```python
from build123d import *

# Parameters (mm, degrees)
SKETCH1_W           = 145
SKETCH1_H           = 43
BOSS_EXTRUDE1_DEPTH = 30
SKETCH2_R           = 3
BOSS_EXTRUDE2_DEPTH = 30


with BuildPart() as part:
    # Sketch1 → Boss-Extrude1 (new body)
    with BuildSketch(Plane(origin=(0, 0, 0), x_dir=(1, 0, 0), z_dir=(0, 1, 0))):
        Rectangle(SKETCH1_W, SKETCH1_H)
    extrude(amount=BOSS_EXTRUDE1_DEPTH)

    # Sketch2 → Boss-Extrude2 (add)
    with BuildSketch(Plane(origin=(72.5, 0, 0), x_dir=(0, 0, -1), z_dir=(1, 0, 0))):
        with Locations((18.5, 25)):
            Circle(SKETCH2_R)
        with Locations((18.5, 5)):
            Circle(SKETCH2_R)
    extrude(amount=BOSS_EXTRUDE2_DEPTH)


solid = part.part
```
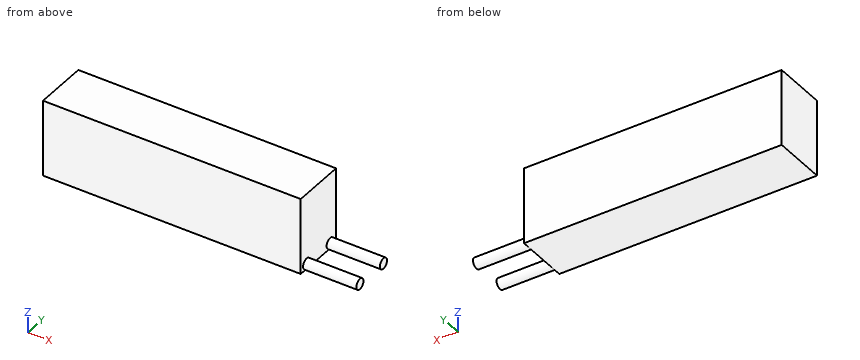
Input: part model. Units: mm. Frame: model coordinates. Give positions to 0.01 mm unless a question says otherwise; leave off trailing zeros. Order: outer loops, then holes, each group sorted by start corner. A loop starts at its lowest first (then second) coordinate and runs counter-clockwise, first axis right, second up. Notation, with made-up numbers: M 7.25,79 L 35.25,79 A21 cw 35.25,85 Z; hole C 11,70 d2. An arc over 180 degrees is marked long. Return JSON: item names as keys, results as strings.
Item 1: First-contact query: P1, Ø12, axis at x = 81, z = -13.5, coming from the -Y side. Flat tip, straight axial feed; report the tip coordinate or a pass-through.
Solutions:
{"P1": "y = 2"}
Item 2: Ray query, probe 1 along X at (y, z) = (15.25, 0); probe 2 along Z at (x, y) = (75, 27). Return the intervals inside material, ascending.
Solutions:
{"probe 1": "-72.5 to 72.5", "probe 2": "-20.74 to -16.26"}
Item 3: Cut plane C-C (z = 9). Return loops of the section in (x, y).
Solutions:
{"outline": "M -72.5,0 L 72.5,0 L 72.5,30 L -72.5,30 Z"}
Item 4: Cut plane A-A (z = -18.5). Return loops of the section in (x, y), then the cut area to 3 significant figures.
Solutions:
{"outline": "M -72.5,0 L 72.5,0 L 72.5,2 L 102.5,2 L 102.5,8 L 72.5,8 L 72.5,22 L 102.5,22 L 102.5,28 L 72.5,28 L 72.5,30 L -72.5,30 Z", "area": "4,710 mm^2"}
Item 5: Cut plane B-B (y = 20). Return loops of the section in (x, z), then the cut area to 4 significant figures.
Solutions:
{"outline": "M -72.5,-21.5 L 72.5,-21.5 L 72.5,21.5 L -72.5,21.5 Z", "area": "6,235 mm^2"}
